from build123d import *

# Parameters (mm, degrees)
F0_R      = 14.55
F1_DEPTH  = 31.5
F2_R      = 13.85
F3_DEPTH  = 15
F4_R      = 5
F5_DEPTH  = 2.3
F6_R      = 1.15
F7_DEPTH  = 22.7
F8_R      = 1.3
F9_DEPTH  = 5
F10_R     = 5
F11_DEPTH = 2.5
F12_W     = 0.5
F12_H     = 2
F13_DEPTH = 4
F16_DEPTH = 10


with BuildPart() as f1:
    # F0 (on Front) → F1 (new body)
    with BuildSketch(Plane.XZ):
        Circle(F0_R)
    extrude(amount=-F1_DEPTH)

    # F2 (on face) → F3 (join)
    with BuildSketch(Plane(origin=(0, 31.5, 0), x_dir=(-1, 0, 0), z_dir=(0, 1, 0))):
        Circle(F2_R)
    extrude(amount=F3_DEPTH)

    # F4 (on face) → F5 (join)
    with BuildSketch(Plane.XZ):
        Circle(F4_R)
    extrude(amount=F5_DEPTH)

    # F6 (on face) → F7 (join)
    with BuildSketch(Plane.XZ.offset(2.3)):
        Circle(F6_R)
    extrude(amount=F7_DEPTH)

    # F8 (on face) → F9 (cut)
    with BuildSketch(Plane.XZ):
        with Locations((0, 8)):
            Circle(F8_R)
        with Locations((0, -8)):
            Circle(F8_R)
    extrude(amount=-F9_DEPTH, mode=Mode.SUBTRACT)

    # F10 (on face) → F11 (join)
    with BuildSketch(Plane(origin=(0, 46.5, 0), x_dir=(-1, 0, 0), z_dir=(0, 1, 0))):
        Circle(F10_R)
    extrude(amount=F11_DEPTH)

    # F12 (on face) → F13 (join)
    with BuildSketch(Plane(origin=(0, 46.5, 0), x_dir=(-1, 0, 0), z_dir=(0, 1, 0))):
        with Locations((-10.25, 0)):
            Rectangle(F12_W, F12_H)
        with Locations((10.25, 0)):
            Rectangle(F12_W, F12_H)
    extrude(amount=F13_DEPTH)

    # F15 (on offset) → F16 (join)
    with BuildSketch(Plane.XZ.offset(7)):
        Polygon((0.15, 0.988686), (0.004988, 0.032877), (0.19347, 0.969916), (0.277389, 1.027876), (0.206972, 1.176383), (0.095135, 1.065977), align=None)
        Polygon((0.317998, 0.942232), (0.009215, 0.026125), (0.357549, 0.916199), (0.450257, 0.958705), (0.406698, 1.117184), (0.277389, 1.027876), align=None)
        Polygon((0.022556, 0.994326), (0.095135, 1.065977), (0, 1.2), (-0.090965, 1.071852), (-0.023513, 1.005262), (-0.000347, 0.038793), align=None)
        Polygon((0.59311, 1.024202), (0.450257, 0.958705), (0.475378, 0.86731), (0.012205, 0.018741), (0.509807, 0.834805), (0.608488, 0.860567), align=None)
        Polygon((-0.15, 0.988686), (-0.090965, 1.071852), (-0.207928, 1.187318), (-0.275259, 1.045321), (-0.197268, 0.991456), (-0.006629, 0.043692), align=None)
        Polygon((0.760543, 0.900263), (0.608488, 0.860567), (0.617356, 0.766199), (0.013868, 0.01095), (0.645618, 0.728209), (0.747273, 0.736444), align=None)
        Polygon((-0.318955, 0.953168), (-0.275259, 1.045321), (-0.410496, 1.138723), (-0.452146, 0.987191), (-0.365986, 0.947687), (-0.013666, 0.047427), align=None)
        Polygon((0.903912, 0.749132), (0.747273, 0.736444), (0.73962, 0.641969), (0.014152, 0.002989), (0.760855, 0.599649), (0.862396, 0.590106), align=None)
        Polygon((-0.524541, 0.875286), (-0.021244, 0.049882), (-0.479176, 0.88885), (-0.452146, 0.987191), (-0.601547, 1.055691), (-0.616251, 0.899228), align=None)
        Polygon((0.838454, 0.498396), (0.01305, -0.004901), (0.852018, 0.453031), (0.950359, 0.426001), (1.018859, 0.575402), (0.862396, 0.590106), align=None)
        Polygon((-0.668114, 0.776452), (-0.029134, 0.050985), (-0.625794, 0.797687), (-0.616251, 0.899228), (-0.775277, 0.940744), (-0.762589, 0.784105), align=None)
        Polygon((0.910855, 0.339841), (0.010595, -0.012479), (0.916335, 0.29281), (1.008489, 0.249114), (1.101891, 0.384351), (0.950359, 0.426001), align=None)
        Polygon((-0.792344, 0.654188), (-0.037095, 0.0507), (-0.754354, 0.68245), (-0.762589, 0.784105), (-0.926408, 0.797376), (-0.886712, 0.64532), align=None)
        Polygon((0.954624, 0.171123), (0.00686, -0.019516), (0.951854, 0.123855), (1.03502, 0.06482), (1.150486, 0.181783), (1.008489, 0.249114), align=None)
        Polygon((-0.893455, 0.51221), (-0.044886, 0.049037), (-0.86095, 0.546639), (-0.886712, 0.64532), (-1.050347, 0.629942), (-0.98485, 0.487089), align=None)
        Polygon((0.96843, -0.002632), (0.001961, -0.025798), (0.957494, -0.048701), (1.029145, -0.12128), (1.163168, -0.026145), (1.03502, 0.06482), align=None)
        Polygon((-0.968377, 0.35483), (-0.05227, 0.046047), (-0.942344, 0.394381), (-0.98485, 0.487089), (-1.143329, 0.44353), (-1.054021, 0.314221), align=None)
        Polygon((0.951854, -0.176145), (-0.003955, -0.031133), (0.933084, -0.219615), (0.991044, -0.303534), (1.13955, -0.233117), (1.029145, -0.12128), align=None)
        Polygon((-1.014831, 0.186832), (-0.059022, 0.04182), (-0.996062, 0.230302), (-1.054021, 0.314221), (-1.202528, 0.243804), (-1.092122, 0.131968), align=None)
        Polygon((0.9054, -0.344143), (-0.010707, -0.03536), (0.879367, -0.383694), (0.921873, -0.476402), (1.080352, -0.432843), (0.991044, -0.303534), align=None)
        Polygon((-1.031407, 0.013319), (-0.064938, 0.036485), (-1.020471, 0.059388), (-1.092122, 0.131968), (-1.226145, 0.036832), (-1.097997, -0.054133), align=None)
        Polygon((0.830478, -0.501523), (-0.018091, -0.03835), (0.797973, -0.535952), (0.823735, -0.634633), (0.98737, -0.619255), (0.921873, -0.476402), align=None)
        Polygon((-1.017601, -0.160436), (-0.069837, 0.030203), (-1.014831, -0.113168), (-1.097997, -0.054133), (-1.213463, -0.171096), (-1.071466, -0.238427), align=None)
        Polygon((0.729367, -0.643501), (-0.025882, -0.040013), (0.691377, -0.671763), (0.699612, -0.773418), (0.863431, -0.786688), (0.823735, -0.634633), align=None)
        Polygon((-0.973832, -0.329154), (-0.073572, 0.023166), (-0.979313, -0.282123), (-1.071466, -0.238427), (-1.164868, -0.373663), (-1.013336, -0.415314), align=None)
        Polygon((0.605137, -0.765765), (-0.033843, -0.040297), (0.562817, -0.787), (0.553274, -0.888541), (0.7123, -0.930057), (0.699612, -0.773418), align=None)
        Polygon((-0.901431, -0.487709), (-0.076027, 0.015588), (-0.914995, -0.442344), (-1.013336, -0.415314), (-1.081836, -0.564715), (-0.925373, -0.579419), align=None)
        Polygon((0.461563, -0.864599), (-0.041733, -0.039195), (0.416199, -0.878163), (0.389169, -0.976504), (0.53857, -1.045004), (0.553274, -0.888541), align=None)
        Polygon((-0.802597, -0.631282), (-0.07713, 0.007698), (-0.823832, -0.588962), (-0.925373, -0.579419), (-0.966889, -0.738445), (-0.81025, -0.725757), align=None)
        Polygon((0.303009, -0.937), (-0.049311, -0.03674), (0.255978, -0.94248), (0.212282, -1.034634), (0.347518, -1.128036), (0.389169, -0.976504), align=None)
        Polygon((-0.680334, -0.755512), (-0.076845, -0.000263), (-0.708595, -0.717522), (-0.81025, -0.725757), (-0.823521, -0.889576), (-0.671465, -0.84988), align=None)
        Polygon((0.134291, -0.980769), (-0.056348, -0.033005), (0.087023, -0.977999), (0.027988, -1.061165), (0.144951, -1.176631), (0.212282, -1.034634), align=None)
        Polygon((-0.538355, -0.856623), (-0.075182, -0.008054), (-0.572784, -0.824118), (-0.671465, -0.84988), (-0.656087, -1.013515), (-0.513234, -0.948018), align=None)
        Polygon((-0.039464, -0.994575), (-0.06263, -0.028106), (-0.085533, -0.983639), (-0.158113, -1.05529), (-0.062977, -1.189313), (0.027988, -1.061165), align=None)
        Polygon((-0.380976, -0.931545), (-0.072192, -0.015438), (-0.420526, -0.905512), (-0.513234, -0.948018), (-0.469675, -1.106497), (-0.340366, -1.017189), align=None)
        Polygon((-0.212977, -0.977999), (-0.067965, -0.02219), (-0.256447, -0.959229), (-0.340366, -1.017189), (-0.269949, -1.165696), (-0.158113, -1.05529), align=None)
    extrude(amount=F16_DEPTH)


solid = f1.part
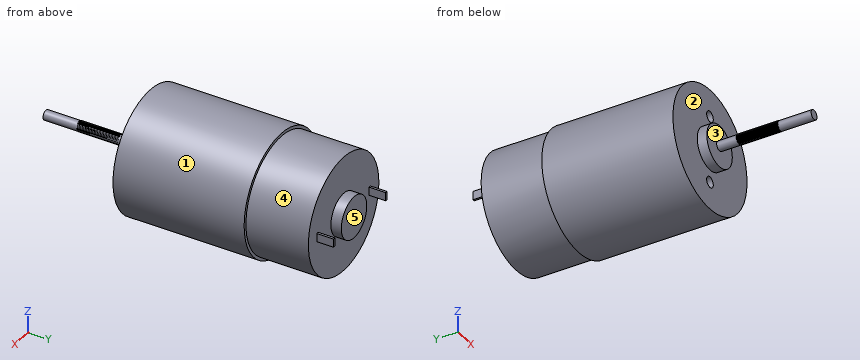
The listing builds one solid part. Answer for the finished solid, in the listing's coordinates (mm). Face numbers are marked on the shaded views. A direction names the side the tool comes from. Coordinates: 2 decimals unless noted, no trailing zeros. Order: outer loops, then holes, each group sorted by start corner. A loop starts at its lowest first (then second) coordinate and runs counter-clockwise, first axis right, second up.
Q1. A cutting plane is placed at D-D, the plane x = 6.75. Write down the section's boundary in (y, z), and give its area (3 significant figures).
Q2. For a pull along X with two mould halves and no side action, classify the marked faces 3, 4 and 5 as pulls with the +X half, pulls with the -X half, needs draft (parallel to the pull), parting line crosses it, or undercut.
Q3. Consider line 1 (Z direction, x = 0, y = 1.9); line 2 (Y direction, x = 3, z = 0); line 3 (Y direction, x = -9, z = -6.5). Determine where each line is inside the solid, lowest interval first.
Q4. Which of the six approach directions +Z, -Z, +X, -X, +Y, -Y give full straight-line access (tool end or side, diameter ignored) to the marked faces 1 and 2?
Q5. Given P1, Ø4, axis at x = 6.5, z = 4, coming from the +Y side; P2, Ø1, axis at y = 49, z = 0.5, coming from the -X side; P3, Ø1, axis at x = 3.5, y = -3.5, coming from the +Z side; P4, Ø12, axis at y = -14, z = -4, coming from the -X side, each flat-ended and moving along its own axis, determine where each tip first touches the part or whether it passes through.
Q6. A cutting plane is placed at C-C, the plane y = 33.5. Write down the section's boundary in (x, z).
Q7. A cutting plane is placed at B-B, the plane z = -8. Write down the section's boundary in (x, y).
Q8. A cutting plane is placed at A-A, the plane x = -7.75. Write down the section's boundary in (y, z).
Answers follow:
1. outline: (0, -12.89) - (31.5, -12.89) - (31.5, -12.09) - (46.5, -12.09) - (46.5, 12.09) - (31.5, 12.09) - (31.5, 12.89) - (0, 12.89) - close
1. area: 1,170 mm2
2. face 3: needs draft
2. face 4: parting line crosses it
2. face 5: undercut
3. line 1: z = -14.55 to -9.3, -6.7 to 6.7, 9.3 to 14.55
3. line 2: y = -2.3 to 49
3. line 3: y = 0 to 46.5
4. face 1: +Y, -Y
4. face 2: -Y
5. P1: stops at y = 46.5
5. P2: stops at x = -10.5
5. P3: passes through
5. P4: stops at x = -1.23
6. outline: circle Ø27.7 at (0, 0)
7. outline: (-12.15, 0) - (-1.3, 0) - (-1.3, 5) - (1.3, 5) - (1.3, 0) - (12.15, 0) - (12.15, 31.5) - (11.31, 31.5) - (11.31, 46.5) - (-11.31, 46.5) - (-11.31, 31.5) - (-12.15, 31.5) - close
8. outline: (0, -12.31) - (31.5, -12.31) - (31.5, -11.48) - (46.5, -11.48) - (46.5, 11.48) - (31.5, 11.48) - (31.5, 12.31) - (0, 12.31) - close
